```python
from build123d import *

# Parameters (mm, degrees)
BASE_DEPTH                     = 6
ESQUISSE3_R                    = 2
ESQUISSE3_W                    = 65
ESQUISSE3_H                    = 30
ENL_V_MAT_EXTRU_1_DEPTH        = 10
CONG_1_R                       = 3
ESQUISSE6_R                    = 2
ESQUISSE6_R_2                  = 10.5
PER_AGE_POUR_BILLES_DEPTH      = 10
PER_AGE_POUR_BILLES_DEPTH_BACK = 10
ESQUISSE8_R                    = 3
PER_AGE_POUR_PROFIL_DEPTH      = 10
PER_AGE_POUR_PROFIL_DEPTH_BACK = 10
ESQUISSE10_R                   = 2
ESQUISSE10_R_2                 = 1.6
ESQUISSE10_R_3                 = 1.625
ENL_V_MAT_EXTRU_3_DEPTH        = 10
ENL_V_MAT_EXTRU_3_DEPTH_BACK   = 10


with BuildPart() as part:
    # Esquisse1 → Base (new body)
    with BuildSketch(Plane.XY):
        Polygon((24.748737342, 24.748737342), (0, 0), (-150, 0), (-174.748737342, 24.748737342), (-174.748737342, 274.748737342), (-150, 299.497474683), (0, 299.497474683), (24.748737342, 274.748737342), align=None)
    extrude(amount=BASE_DEPTH)

    # Esquisse3 → Enlèv. mat.-Extru.1 (cut)
    with BuildSketch(Plane(origin=(0, 0, 0), x_dir=(-1, 0, 0), z_dir=(0, 0, -1))):
        with Locations((40, 45)):
            Circle(ESQUISSE3_R)
        with Locations((110, 45)):
            Circle(ESQUISSE3_R)
        with Locations((110, 254.497474683)):
            Circle(ESQUISSE3_R)
        with Locations((40, 254.497474683)):
            Circle(ESQUISSE3_R)
        Polygon((117, 0), (117, 20), (93, 20), (93, 45.5), (57, 45.5), (57, 20), (33, 20), (33, 0), align=None)
        Polygon((33, 299.497474683), (117, 299.497474683), (117, 279.497474683), (93, 279.497474683), (93, 253.997474683), (57, 253.997474683), (57, 279.497474683), (33, 279.497474683), align=None)
        with Locations((75, 229.497474683)):
            Rectangle(ESQUISSE3_W, ESQUISSE3_H)
        with Locations((75, 70)):
            Rectangle(ESQUISSE3_W, ESQUISSE3_H)
    extrude(amount=-ENL_V_MAT_EXTRU_1_DEPTH, mode=Mode.SUBTRACT)

    # Congé1
    cong_1_edges = [part.edges().sort_by_distance(p)[0] for p in [
        (-117, 0, 3),
        (-33, 0, 3),
        (-33, 20, 3),
        (-57, 20, 3),
        (-57, 45.5, 3),
        (-93, 45.5, 3),
        (-93, 20, 3),
        (-117, 20, 3),
        (0, 0, 3),
        (-150, 0, 3),
        (-174.748737342, 24.748737342, 3),
        (-174.748737342, 274.748737342, 3),
        (-150, 299.497474683, 3),
        (0, 299.497474683, 3),
        (24.748737342, 274.748737342, 3),
        (24.748737342, 24.748737342, 3),
        (-33, 279.497474683, 3),
        (-33, 299.497474683, 3),
        (-117, 299.497474683, 3),
        (-117, 279.497474683, 3),
        (-93, 279.497474683, 3),
        (-93, 253.997474683, 3),
        (-57, 253.997474683, 3),
        (-57, 279.497474683, 3),
    ]]
    fillet(cong_1_edges, radius=CONG_1_R)

    # Esquisse6 → Perçage pour billes (cut, two sides)
    with BuildSketch(Plane.XY.offset(5)) as per_age_pour_billes_sk:
        with Locations((-152, 55)):
            Circle(ESQUISSE6_R)
        with Locations((-152, 85)):
            Circle(ESQUISSE6_R)
        with Locations((-152, 70)):
            Circle(ESQUISSE6_R_2)
        with Locations((-152, 244.497474683)):
            Circle(ESQUISSE6_R)
        with Locations((-152, 214.497474683)):
            Circle(ESQUISSE6_R)
        with Locations((-152, 229.497474683)):
            Circle(ESQUISSE6_R_2)
        with Locations((-20.251262658, 259.497474683)):
            Circle(ESQUISSE6_R)
        with Locations((-5.251262658, 259.497474683)):
            Circle(ESQUISSE6_R_2)
        with Locations((9.748737342, 259.497474683)):
            Circle(ESQUISSE6_R)
        with Locations((9.748737342, 40)):
            Circle(ESQUISSE6_R)
        with Locations((-5.251262658, 40)):
            Circle(ESQUISSE6_R_2)
        with Locations((-20.251262658, 40)):
            Circle(ESQUISSE6_R)
    extrude(amount=PER_AGE_POUR_BILLES_DEPTH, mode=Mode.SUBTRACT)
    extrude(per_age_pour_billes_sk.sketch, amount=-PER_AGE_POUR_BILLES_DEPTH_BACK, mode=Mode.SUBTRACT)

    # Esquisse8 → Perçage pour profilé (cut, two sides)
    with BuildSketch(Plane.XY.offset(5)) as per_age_pour_profil_sk:
        with Locations((-133, 16)):
            Circle(ESQUISSE8_R)
        with Locations((-133, 283.497474683)):
            Circle(ESQUISSE8_R)
        with Locations((-17, 283.497474683)):
            Circle(ESQUISSE8_R)
        with Locations((-17, 16)):
            Circle(ESQUISSE8_R)
    extrude(amount=PER_AGE_POUR_PROFIL_DEPTH, mode=Mode.SUBTRACT)
    extrude(per_age_pour_profil_sk.sketch, amount=-PER_AGE_POUR_PROFIL_DEPTH_BACK, mode=Mode.SUBTRACT)

    # Esquisse10 → Enlèv. mat.-Extru.3 (cut, two sides)
    with BuildSketch(Plane.XY.offset(5)) as enl_v_mat_extru_3_sk:
        with Locations((-108, 204.497474683)):
            Circle(ESQUISSE10_R)
        with Locations((-108, 177.997474683)):
            Circle(ESQUISSE10_R)
        with Locations((-42, 177.997474683)):
            Circle(ESQUISSE10_R)
        with Locations((-42, 204.497474683)):
            Circle(ESQUISSE10_R)
        with Locations((-42, 121.5)):
            Circle(ESQUISSE10_R)
        with Locations((-42, 95)):
            Circle(ESQUISSE10_R)
        with Locations((-108, 121.5)):
            Circle(ESQUISSE10_R)
        with Locations((-108, 95)):
            Circle(ESQUISSE10_R)
        with Locations((-28.5, 176.748737342)):
            Circle(ESQUISSE10_R_2)
        with Locations((-28.5, 122.748737342)):
            Circle(ESQUISSE10_R_2)
        with Locations((-168.498737342, 179.748737342)):
            Circle(ESQUISSE10_R_2)
        with Locations((-168.498737342, 119.748737342)):
            Circle(ESQUISSE10_R_2)
        with Locations((-18.251262658, 149.748737342)):
            Circle(ESQUISSE10_R_3)
        with Locations((9.748737342, 149.748737342)):
            Circle(ESQUISSE10_R_3)
        with Locations((9.748737342, 72.748737342)):
            Circle(ESQUISSE10_R_3)
        with Locations((9.748737342, 226.748737342)):
            Circle(ESQUISSE10_R_3)
        with Locations((-18.251262658, 72.748737342)):
            Circle(ESQUISSE10_R_3)
        with Locations((-18.251262658, 226.748737342)):
            Circle(ESQUISSE10_R_3)
    extrude(amount=ENL_V_MAT_EXTRU_3_DEPTH, mode=Mode.SUBTRACT)
    extrude(enl_v_mat_extru_3_sk.sketch, amount=-ENL_V_MAT_EXTRU_3_DEPTH_BACK, mode=Mode.SUBTRACT)


solid = part.part
```
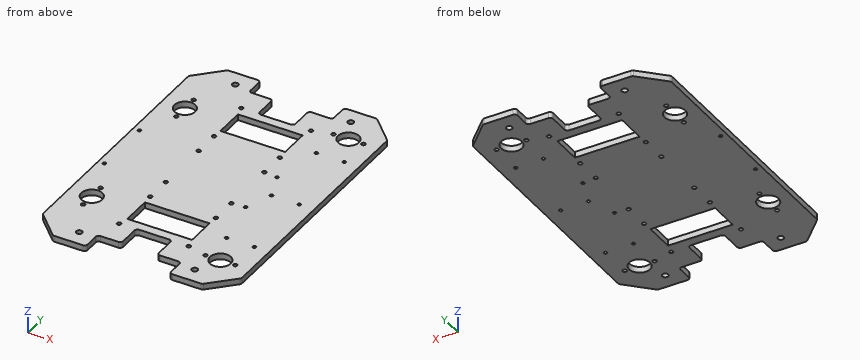
Geometry: final body of the model. Coordinates: model frame, mm. Give positions to 0.01 mm unless a question says otherwise; leave off trailing zeros. Order: outer loops, then holes, each group sorted by start corner. A loop starts at its lowest first (then second) coordinate and runs counter-clockwise, first axis right, second up. Notation, with made-up numbers: M -31.75,38.5 L -8.75,38.5 A13 ccw -8.75,53.5 Z; hole C -23,63.5 d1. An arc over 180 degrees is marked long. Answer as CSV lines item,"result". Start each with the question number.
1) Cut plane B-B (z = 4.7). State how many separate pieces and enclosed holes the cut face has, then the cut area to 3 significant figures.
2) First-contact query: P1, Ø3, axis at x = -18.25, y = 149.75, coming from the +Z side; P2, Ø1, axis at x = -54.5, z = 5, coming from the +Y side; P3, Ø2, axis at x = -76.5, z = 4, coming from the -Y side. Flat tips, straight axial feed; report the tip coordinate or a pass-through.
3) Line query: line 1 (Y direction, x = -48, z = 0.7); line 2 (X direction, y = 40, z = 4.55); line 3 (Y direction, x = -11, z = 0.65). Output: solid intervals per line, ascending. Write a range as from..to.
4) Cut plane A-A (x = -158). Output: boundary loops of the cut face in (y, z).
Findings below:
1,separate pieces,"1"
1,enclosed holes,"40"
1,area,"47,600 mm²"
2,P1,"passes through"
2,P2,"stops at y = 279.5"
2,P3,"stops at y = 45.5"
3,line 1,"y = 20..55, 85..214.5, 244.5..279.5"
3,line 2,"x = -174.75..-93, -57..-22.25, -18.25..-15.75, 5.25..7.75, 11.75..24.75"
3,line 3,"y = 0..31.21, 48.79..250.71, 268.28..299.5"
4,outline,"M 8,0 L 61.38,0 L 61.38,6 L 8,6 Z; M 78.62,0 L 220.88,0 L 220.88,6 L 78.62,6 Z; M 238.11,0 L 291.5,0 L 291.5,6 L 238.11,6 Z"
